Part model, mm, in its own coordinate system. Give positions to 0.01 mm unless a question says otherwise; leave off trailing zeros. Order: outer loops, then holes, each group sorted by start corner. A loop starts at its lowest first (then second) coordinate and runs counter-clockwise, first axis right, second up. Notation, with made-up numbers: (78, 38) -> (106, 38) arc R9 cw to (106, 48) -> close; hole circle Ø10 at (47.25, 73.5). An arc over 180 degrees is marked (long way). Write item = value, one per line. Start each with the question number.
(1) Saw through at A-A, the plane z = 0. List the corners of the cut face in (x, y).
(2) Saw through at B-B, the plane y = 234. List the corners of the cut face in (x, z).
(3) Flat gauge pins, fed straight in: pin 1 (3 mm diameter, centred on x = -100, z = 4, fed in from +Y); pin 2 (1 mm diameter, centred on y = 936.5, z = -1, fed in from +X); pin 3 (8 mm diameter, centred on y = 867, z = 1, fed in from -X). Where does each tip first touch, or does it go through?
(4) Probe line 1 along X through (y, z) = (1260, 0.75); line 2 along X through (y, z) = (1261, -2); line 3 along Y through (x, z) = (-120, 5.25). List the from-to ranges inside material, lowest first. Write a range as from..to.
from build123d import *

# Parameters (mm, degrees)
SKETCH_2_R = 7.5


with BuildPart() as part:
    # 扫描1: sweep along a path in 草图1
    with BuildLine(Plane.XY) as sweep_1_path:
        Line((-132.24, 1375.12), (-132.24, 1195.025238859))
        ThreePointArc((-132.24, 1195.025238859), (-131.214906225, 1186.027645585), (-128.192165763, 1177.491221153))
        ThreePointArc((-128.192165763, 1177.491221153), (-119.60577967, 1161.723839886), (-109.64, 1146.79))
        ThreePointArc((-109.64, 1146.79), (-90.212182039, 1121.745991014), (-69.488938494, 1097.76287875))
        ThreePointArc((-69.488938494, 1097.76287875), (-41.828906751, 1067.358377322), (-14.221130337, 1036.906419346))
        ThreePointArc((-14.221130337, 1036.906419346), (-3.678280273, 1019.775770131), (0, 1000))
        Line((0, 1000), (0, 0))
    # 草图2 → 扫描1 (sweep)
    with BuildSketch(Plane(origin=(0, 0, 0), x_dir=(1, 0, 0), z_dir=(0, 1, 0))):
        Circle(SKETCH_2_R)
    sweep(path=sweep_1_path.line)


solid = part.part
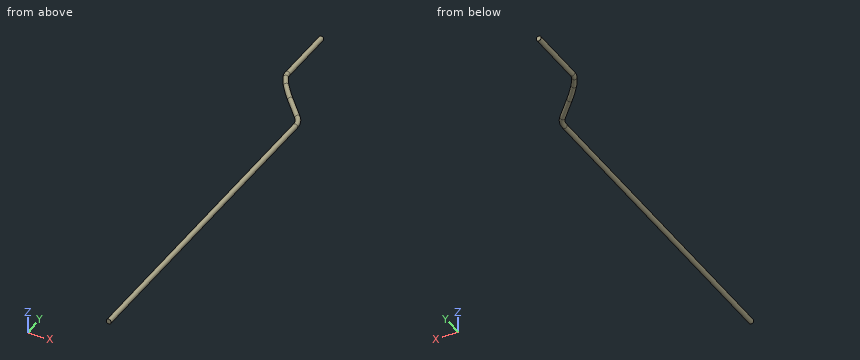
Results list:
q1.outline = (-139.74, 1195.03) arc R47.5 ccw to (-134.93, 1174.2) arc R207.5 ccw to (-115.69, 1142.35) arc R607.5 ccw to (-75.03, 1092.71) arc R23927.13 cw to (-19.78, 1031.87) arc R47.5 cw to (-7.5, 1000) -> (-7.5, 0) -> (7.5, 0) -> (7.5, 1000) arc R62.5 ccw to (-8.66, 1041.94) arc R23942.13 ccw to (-63.95, 1102.81) arc R592.5 cw to (-103.59, 1151.23) arc R192.5 cw to (-121.45, 1180.78) arc R32.5 cw to (-124.74, 1195.03) -> (-124.74, 1375.12) -> (-139.74, 1375.12) -> close
q2.outline = circle Ø15 at (0, 0)
q3.pin_1 = 1146.88
q3.pin_2 = 7.48
q3.pin_3 = -7.5
q4.line_1 = -139.7..-124.78
q4.line_2 = -139.47..-125.01
q4.line_3 = 1152.31..1173.23
